Work out the finished part from the listing and answer in its coordinate system (mm). A direction names the side the tool comes from. Coordinates: 2 decimals unless noted, no trailing zeros. Order: outer loops, then holes, each group sorted by start corner. A loop starts at its lowest first (then second) coordinate and runs counter-clockwise, first axis right, second up. Notation, with made-up numbers: M 83,37.5 L 107,37.5 A32 ccw 107,63.5 Z; hole C -10,57 d7. An arc over 180 degrees is marked long. Use a Markdown table: item, result.
from build123d import *


with BuildPart() as part:
    # Sketch1 → Revolve1 (revolve)
    with BuildSketch(Plane.XY, mode=Mode.PRIVATE) as revolve1_sk:
        Polygon((-40.878125000000004, 14.684375), (40.87812500000002, 14.68437500000001), (40.878125000000026, -5.3e-15), (-40.87812500000002, -1.531e-14), align=None)
    revolve(revolve1_sk.sketch.rotate(Axis((0, 0, 0), (1, 0, 0)), 90), axis=Axis((0, 0, 0), (1, 0, 0)))

    # Sketch2 → Revolve2 (revolve)
    with BuildSketch(Plane.XY, mode=Mode.PRIVATE) as revolve2_sk:
        Polygon((-35.91760263939639, 26.660135359424125), (1.125953860013809, -10.383421139986174), (11.509375000000016, 0), (-25.53418149941018, 37.043556499410315), align=None)
    revolve(revolve2_sk.sketch.rotate(Axis((-22.918474439856404, 34.427849439856544, 0), (-0.7071067811865464, 0.7071067811865488, 0)), 180), axis=Axis((-22.918474439856404, 34.427849439856544, 0), (-0.7071067811865464, 0.7071067811865488, 0)))

    # Sketch3 → Cut-Revolve1 (revolve, cut)
    with BuildSketch(Plane.XY):
        Polygon((-25.534181499651336, 37.043556499169185), (-33.0775966413494, 29.500141357471097), (-17.362148429478385, 13.784693145600082), (-15.40445259508532, 15.742388979993137), (5.92365569245394, -5.585719307546082), (11.509375000000016, 0), align=None)
    revolve(axis=Axis((-25.534181499651336, 37.043556499169185, 0), (0.707106781186548, -0.707106781186547, 0)), mode=Mode.SUBTRACT)

    # Sketch4 → Cut-Revolve2 (revolve, cut)
    with BuildSketch(Plane.XY, mode=Mode.PRIVATE) as cut_revolve2_sk:
        Polygon((40.87812500000001, 10.667999999999994), (17.85937500000001, 10.667999999999994), (17.85937500000001, 7.899399999999997), (-18.653124999999985, 7.89939999999999), (-18.653124999999985, 10.667999999999987), (-40.87812500000002, 10.667999999999983), (-40.87812500000002, -1.531e-14), (40.878125000000026, -5.3e-15), align=None)
    revolve(cut_revolve2_sk.sketch.rotate(Axis((17.859375000000455, 0, 0), (-1, 0, 0)), 90), axis=Axis((17.859375000000455, 0, 0), (-1, 0, 0)), mode=Mode.SUBTRACT)


solid = part.part
1. Section B-B on y = -5 is taken. Determine the outline of the cut face in (x, z).
Answers below:
| item | result |
|---|---|
| outline | M -40.88,-13.81 L 40.88,-13.81 L 40.88,-9.42 L 17.86,-9.42 L 17.86,-6.12 L -18.65,-6.12 L -18.65,-9.42 L -40.88,-9.42 Z; M -40.88,9.42 L -18.65,9.42 L -18.65,6.12 L 17.86,6.12 L 17.86,9.42 L 40.88,9.42 L 40.88,13.81 L -40.88,13.81 Z |
2. For a pull along Y with two mould halves and no side action, classify faces 6 (the face through (-0.965, 32.282, -4.411)), 7 (the face through (-20.1, 42.48, -7.68)), 8 (the face through (-40.878, -8, -8)) as +Y half, -Y half, draft (parallel to the pull), parting line (faces both ways), or undercut.
Answers below:
| item | result |
|---|---|
| face 6 | undercut |
| face 7 | +Y half |
| face 8 | draft |
3. Flat-ended cylindrical pins translate along their axes: P1, Ø3, axis at x = -4.5, z = 5, coming from the +Y side; P2, Ø4, axis at x = -10.5, y = -6, coming from the +Z side; P3, Ø1.5, axis at x = -21.5, y = -8, coming from the -Z side. Find the tip coordinate at first contact, or state that the pin passes through.
Answers below:
| item | result |
|---|---|
| P1 | y = 37.2 |
| P2 | z = 14.13 |
| P3 | z = -12.77 |
4. For faces 1 (the face through (-0.65, -7.83, 1.03)), 2 (the face through (-18.653, 4, -7)), 3 (the face through (40.878, -8, 8)), 4 (the face through (0.57, -14.56, -1.91)), 5 (the face through (17.859, 4, 7)), determine the directions among +Z, -Z, +X, -X, +Y, -Y from which every point of the face is accessible in a straight line to the end or side of a thin tool.
Answers below:
| item | result |
|---|---|
| face 1 | +X, -X |
| face 2 | -X |
| face 3 | +Z, -Z, +X, +Y, -Y |
| face 4 | none |
| face 5 | +X |
5. Section D-D on z = 6.25 is taken. Determine the outline of the cut face in (x, y).
Answers below:
| item | result |
|---|---|
| outline | M -40.88,-13.29 L 40.88,-13.29 L 40.88,-8.65 L 17.86,-8.65 L 17.86,-4.83 L -18.65,-4.83 L -18.65,-8.65 L -40.88,-8.65 Z; M -40.88,8.65 L -18.65,8.65 L -18.65,4.83 L -0.15,4.83 L -13.23,17.91 L -15.93,15.21 L -31.65,30.93 L -34.93,27.65 L -20.57,13.29 L -40.88,13.29 Z; M -19.42,43.16 L -3.71,27.44 L -6.4,24.74 L 13.51,4.83 L 17.86,4.83 L 17.86,8.65 L 40.88,8.65 L 40.88,13.29 L 17.01,13.29 L -16.14,46.44 Z |
6. Section A-A on z = 0 is taken. Determine the outline of the cut face in (x, y), then the cut area to 3 significant figures.
Answers below:
| item | result |
|---|---|
| outline | M -40.88,-14.68 L 40.88,-14.68 L 40.88,-10.67 L 17.86,-10.67 L 17.86,-7.9 L -18.65,-7.9 L -18.65,-10.67 L -40.88,-10.67 Z; M -40.88,10.67 L -18.65,10.67 L -18.65,7.9 L -7.56,7.9 L -15.4,15.74 L -17.36,13.78 L -33.08,29.5 L -35.92,26.66 L -23.94,14.68 L -40.88,14.68 Z; M -17.99,44.59 L -2.28,28.87 L -4.23,26.91 L 14.78,7.9 L 17.86,7.9 L 17.86,10.67 L 40.88,10.67 L 40.88,14.68 L 17.59,14.68 L -15.15,47.43 Z |
| area | 1,010 mm² |
7. Find the intervals of material crossed by probe 1 along X at (y, z) = (16, -4.5); probe 2 along Y at (x, z) = (-11, -3.75); probe 3 along Y at (x, z) = (-35, 1.25), in increasing order.
Answers below:
| item | result |
|---|---|
| probe 1 | -24.26 to -18.17, -15.15 to -13.67, 4.69 to 15.28 |
| probe 2 | -14.2 to -6.95, 6.95 to 12.68, 36.63 to 42.59 |
| probe 3 | -14.63 to -10.59, 10.59 to 14.63, 25.82 to 27.58 |
8. Section C-C on x = 23.5 is taken. Determine the outline of the cut face in (y, z).
Answers below:
| item | result |
|---|---|
| outline | C 0,0 d29.37; hole C 0,0 d21.34 |
